```python
from build123d import *

# Parameters (mm, degrees)
SKETCH1_R                = 18.5
BOSS_EXTRUDE1_DEPTH      = 5
SKETCH2_R                = 6.2
CUT_EXTRUDE1_DEPTH       = 10
SKETCH3_R                = 1.6999999999999995
SKETCH3_R_2              = 1.6999999999998752
SKETCH3_R_3              = 1.7000000000002367
SKETCH3_R_4              = 1.700000000000381
SKETCH3_R_5              = 1.7000000000003195
SKETCH3_R_6              = 1.7000000000003193
CUT_EXTRUDE2_DEPTH       = 10
BOSS_EXTRUDE2_DEPTH      = 50
BOSS_EXTRUDE3_DEPTH      = 7
CUT_EXTRUDE3_DEPTH       = 20
BOSS_EXTRUDE4_DEPTH      = 8.5
BOSS_EXTRUDE4_DEPTH_BACK = 15.499999999999996
SKETCH7_R                = 3.799999999999999
SKETCH8_R                = 4.000000000000005
SKETCH8_R_2              = 1.7500000000000004
SKETCH8_R_3              = 4.000000000000007
BOSS_EXTRUDE5_DEPTH      = 4
CUT_EXTRUDE4_START       = -2
SKETCH8_2_R              = 1.7500000000000004
CUT_EXTRUDE4_DEPTH       = 2
FILLET1_R                = 5
SKETCH9_R                = 3.0000000000000036
CUT_EXTRUDE5_DEPTH       = 2.5
CUT_EXTRUDE6_DEPTH       = 182.00138122207798
FILLET2_R                = 10
SKETCH11_W               = 22.00000000000001
SKETCH11_H               = 61.99999999999998
CUT_EXTRUDE7_DEPTH       = 182.00138122207798
FILLET3_R                = 5


with BuildPart() as part:
    # Sketch1 → Boss-Extrude1 (new body)
    with BuildSketch(Plane(origin=(0, 0, 0), x_dir=(0, 0, -1), z_dir=(1, 0, 0))):
        Circle(SKETCH1_R)
    extrude(amount=BOSS_EXTRUDE1_DEPTH)

    # Sketch2 → Cut-Extrude1 (cut)
    with BuildSketch(Plane(origin=(5, 0, 0), x_dir=(0, 0, -1), z_dir=(1, 0, 0))):
        with Locations((0, 7)):
            Circle(SKETCH2_R)
    extrude(amount=-CUT_EXTRUDE1_DEPTH, mode=Mode.SUBTRACT)

    # Sketch3 → Cut-Extrude2 (cut)
    with BuildSketch(Plane(origin=(0, 0, 0), x_dir=(0, 0, -1), z_dir=(1, 0, 0))):
        with Locations((15.5, 0)):
            Circle(SKETCH3_R)
        with Locations((7.750000000000335, -13.423393758658609)):
            Circle(SKETCH3_R_2)
        with Locations((-7.749999999999674, -13.423393758658612)):
            Circle(SKETCH3_R_3)
        with Locations((-15.499999999999568, 0)):
            Circle(SKETCH3_R_4)
        with Locations((-7.749999999999682, 13.42339375865861)):
            Circle(SKETCH3_R_5)
        with Locations((7.749999999999989, 13.42339375865842)):
            Circle(SKETCH3_R_6)
    extrude(amount=CUT_EXTRUDE2_DEPTH, mode=Mode.SUBTRACT)

    # Sketch4 → Boss-Extrude2 (add)
    with BuildSketch(Plane.ZY):
        with BuildLine():
            Line((-18.5, 0), (-21.5, 0))
            ThreePointArc((-21.5, 0), (-3.95e-15, -21.5), (21.5, 0))
            Line((21.5, 0), (18.5, 0))
            ThreePointArc((18.5, 0), (-3.4e-15, -18.5), (-18.5, 0))
        make_face()
    extrude(amount=-BOSS_EXTRUDE2_DEPTH)

    # Sketch5 → Boss-Extrude3 (add)
    with BuildSketch(Plane.ZY):
        with BuildLine():
            Line((-21.5, 0), (-18.5, 0))
            ThreePointArc((-18.5, 0), (-3.4e-15, -18.5), (18.5, 0))
            Line((18.5, 0), (21.5, 0))
            Line((21.5, 0), (21.500000000000018, -174.5))
            Line((21.500000000000018, -174.5), (-21.49999999999998, -174.5))
            Line((-21.49999999999998, -174.5), (-21.5, 0))
        make_face()
    extrude(amount=-BOSS_EXTRUDE3_DEPTH)

    # Sketch6 → Cut-Extrude3 (cut)
    with BuildSketch(Plane(origin=(7, 0, 0), x_dir=(0, 0, -1), z_dir=(1, 0, 0))):
        with BuildLine():
            ThreePointArc((2.57571e-12, -174.5), (-15.202795795509834, -168.2027957955117), (-21.499999999999957, -153.00000000000003))
            Line((-21.500000000000014, -153.00000000000003), (-21.500000000000018, -174.5))
            Line((-21.500000000000018, -174.5), (2.57572e-12, -174.5))
        make_face()
        with BuildLine():
            Line((21.49999999999998, -174.5), (21.499999999999982, -153.00000000000003))
            ThreePointArc((21.5, -153.00000000000003), (15.20279579551168, -168.20279579550987), (2.57571e-12, -174.5))
            Line((2.57572e-12, -174.5), (21.499999999999982, -174.5))
        make_face()
    extrude(amount=-CUT_EXTRUDE3_DEPTH, mode=Mode.SUBTRACT)

    # Sketch7 → Boss-Extrude4 (add, two sides: drawn at the far end of the back side and taken through both)
    with BuildSketch(Plane(origin=(7, 0, 0), x_dir=(0, 0, -1), z_dir=(1, 0, 0)).offset(-BOSS_EXTRUDE4_DEPTH_BACK)):
        with Locations((2.082e-14, -153.00000000000003)):
            Circle(SKETCH7_R)
    extrude(amount=BOSS_EXTRUDE4_DEPTH + BOSS_EXTRUDE4_DEPTH_BACK)

    # Sketch8 → Boss-Extrude5 (add)
    # profile 1 of 4: a face of its own
    with BuildSketch(Plane(origin=(7, 0, 0), x_dir=(0, 0, -1), z_dir=(1, 0, 0))):
        with Locations(Location((10.160000000000018, -121.88999999999999, 0), (0, 0, 180))):
            Circle(SKETCH8_R)
        with Locations((10.160000000000018, -121.88999999999999)):
            Circle(SKETCH8_R_2, mode=Mode.SUBTRACT)
    # profile 2 of 4: a face of its own
    with BuildSketch(Plane(origin=(7, 0, 0), x_dir=(0, 0, -1), z_dir=(1, 0, 0))):
        with Locations(Location((-10.159999999999984, -121.88999999999999, 0), (0, 0, 180))):
            Circle(SKETCH8_R_3)
        with Locations((-10.159999999999984, -121.88999999999999)):
            Circle(SKETCH8_R_2, mode=Mode.SUBTRACT)
    # profile 3 of 4: a face of its own
    with BuildSketch(Plane(origin=(7, 0, 0), x_dir=(0, 0, -1), z_dir=(1, 0, 0))):
        with Locations(Location((-10.159999999999984, -104.10999999999999, 0), (0, 0, 180))):
            Circle(SKETCH8_R_3)
        with Locations((-10.159999999999984, -104.10999999999999)):
            Circle(SKETCH8_R_2, mode=Mode.SUBTRACT)
    # profile 4 of 4: a face of its own
    with BuildSketch(Plane(origin=(7, 0, 0), x_dir=(0, 0, -1), z_dir=(1, 0, 0))):
        with Locations(Location((10.160000000000018, -104.10999999999999, 0), (0, 0, 180))):
            Circle(SKETCH8_R)
        with Locations((10.160000000000018, -104.10999999999999)):
            Circle(SKETCH8_R_2, mode=Mode.SUBTRACT)
    extrude(amount=BOSS_EXTRUDE5_DEPTH)

    # Sketch8_2 → Cut-Extrude4 (cut)
    with BuildSketch(Plane(origin=(7, 0, 0), x_dir=(0, 0, -1), z_dir=(1, 0, 0)).offset(CUT_EXTRUDE4_START)):
        with Locations((-10.159999999999984, -121.88999999999999)):
            Circle(SKETCH8_2_R)
        with Locations((-10.159999999999984, -104.10999999999999)):
            Circle(SKETCH8_2_R)
        with Locations((10.160000000000018, -104.10999999999999)):
            Circle(SKETCH8_2_R)
        with Locations((10.160000000000018, -121.88999999999999)):
            Circle(SKETCH8_2_R)
    extrude(amount=CUT_EXTRUDE4_DEPTH, mode=Mode.SUBTRACT)

    # Fillet1
    fillet1_edges = [part.edges().sort_by_distance(p)[0] for p in [
        (7, -21.5, -2.2e-15),
    ]]
    fillet(fillet1_edges, radius=FILLET1_R)

    # Sketch9 → Cut-Extrude5 (cut)
    with BuildSketch(Plane(origin=(15.5, 0, 0), x_dir=(0, 0, -1), z_dir=(1, 0, 0))):
        with Locations((2.082e-14, -153.00000000000003)):
            Circle(SKETCH9_R)
    extrude(amount=-CUT_EXTRUDE5_DEPTH, mode=Mode.SUBTRACT)

    # Sketch10 → Cut-Extrude6 (cut, through all)
    with BuildSketch(Plane(origin=(7, 0, 0), x_dir=(0, 0, -1), z_dir=(1, 0, 0))):
        with BuildLine():
            Line((-15.000000000000016, -137.57296518391348), (-15.000000000000014, -21.84605227495347))
            ThreePointArc((-15.000000000000018, -21.84605227495347), (-18.524475882395627, -18.94977026991469), (-21.5, -15.491933384829668))
            Line((-21.5, -15.491933384829668), (-21.5, -152.13779166279446))
            ThreePointArc((-21.500000000000007, -152.13779166279446), (-19.64932677192729, -144.23088598393383), (-15.000000000000014, -137.57296518391348))
        make_face()
        with BuildLine():
            ThreePointArc((21.499999999999996, -15.491933384829675), (18.52447588239562, -18.949770269914705), (14.999999999999996, -21.846052274953482))
            Line((14.999999999999996, -21.846052274953482), (14.999999999999995, -137.57296518391342))
            ThreePointArc((14.999999999999995, -137.57296518391342), (19.649326771927107, -144.23088598393335), (21.499999999999993, -152.1377916627935))
            Line((21.499999999999996, -152.1377916627935), (21.499999999999996, -15.491933384829672))
        make_face()
    extrude(amount=-CUT_EXTRUDE6_DEPTH, mode=Mode.SUBTRACT)

    # Fillet2
    fillet2_edges = [part.edges().sort_by_distance(p)[0] for p in [
        (3.5, -137.57296518391348, 15.000000000000014),
        (3.5, -137.57296518391342, -14.999999999999991),
        (3.5, -21.846052274953486, -14.999999999999998),
        (3.5, -15.491933384829675, -21.5),
        (3.5, -21.846052274953465, 15.000000000000014),
        (3.5, -15.491933384829668, 21.5),
    ]]
    fillet(fillet2_edges, radius=FILLET2_R)

    # Sketch11 → Cut-Extrude7 (cut, through all)
    with BuildSketch(Plane(origin=(7, 0, 0), x_dir=(0, 0, -1), z_dir=(1, 0, 0))):
        with Locations((-8.88e-15, -61.47322598734716)):
            Rectangle(SKETCH11_W, SKETCH11_H)
    extrude(amount=-CUT_EXTRUDE7_DEPTH, mode=Mode.SUBTRACT)

    # Fillet3
    fillet3_edges = [part.edges().sort_by_distance(p)[0] for p in [
        (3.5, -30.47322598734717, -10.999999999999996),
        (3.5, -92.47322598734716, -10.999999999999996),
        (3.5, -92.47322598734716, 11.000000000000014),
        (3.5, -30.47322598734717, 11.000000000000014),
    ]]
    fillet(fillet3_edges, radius=FILLET3_R)


solid = part.part
```
The model under review builds one solid part; all positions refer to its coordinate system, in mm. A direction names the side the tool comes from. Round coordinates to 2 decimals unless told otherwise and drop trailing zeros. Order: outer loops, then holes, each group sorted by start corner. A loop starts at its lowest first (then second) coordinate and runs counter-clockwise, first axis right, second up.
Item 1: Machinability: for faces 4 (the cylindrical face through (3.451, -136.98, 15.516)), 5 (the flat face through (4, -92.473, 0)), 6 (the flat face through (11, -102, 11)), 7 (the flat face through (50, -19, 0)), 8 (the flat face through (5, -122, 10)), which of the approach directions +Z, -Z, +X, -X, +Y, -Y give a long, thin tool a straight path to every point of the face, cutting with its end or side? Answer none if there is none.
Working result:
face 4: +Z, +X, -X
face 5: +X, -X
face 6: +Z, -Z, +X, -Y
face 7: +Z, -Z, +X, +Y, -Y
face 8: +X
Item 2: Add section C-C, the plane y = 5. State the section outline as (x, z) points, and give its area (3 significant figures).
Working result:
outline: (0, -17.81) - (5, -17.81) - (5, -5.87) - (0, -5.87) - close; (0, 5.87) - (5, 5.87) - (5, 17.81) - (0, 17.81) - close
area: 119 mm2
Item 3: Draft analysis for pull direction Y (two halves, no side actions). For faces 1 (the cylindrical face through (-4.31, -156.71, 0.82)), 2 (the flat face through (11, -102, -9)), 3 (the cylindrical face through (2.465, -14.075, 6.18)), state which applies: released by +Y, released by -Y, zero draft, split by the parting line, or undercut.
Working result:
face 1: split by the parting line
face 2: zero draft
face 3: undercut
Item 4: For pin 1 (6.5 mm diameter, centred on y = -153, z = -0.5, fed in from +X); pin 2 (6 mm diameter, centred on x = 10.5, z = 10.5, fed in from -Y); pin 3 (1.5 mm diameter, centred on y = -110.5, z = 3.5, fed in from +X), all flat-tipped, find the tip position at first contact; note any pin that passes through.
Working result:
pin 1: stops at x = 15.5
pin 2: stops at y = -125.89
pin 3: stops at x = 7
Item 5: Add section B-B, the plane z = 0. Count the separate pieces of the cut face and the enclosed holes in it, and give its area (3 significant figures).
Working result:
separate pieces: 3
enclosed holes: 0
area: 1,030 mm2
Item 6: To check wall thickness, follow probe 1 along Y at (x, z) = (14.75, 0); probe 2 along Y at (x, z) = (3.05, 7.75); probe 3 along Y at (x, z) = (3, 7). State the ranges of each line that lie inside material, in increasing order.
Working result:
probe 1: y = -156.8 to -156, -150 to -149.2, -21.5 to -18.5
probe 2: y = -173.05 to -92.16, -30.79 to -15.12, -11.72 to 11.72, 15.12 to 16.8
probe 3: y = -173.33 to -92.37, -30.57 to -14.95, -11.9 to 11.9, 14.95 to 17.12
Item 7: Add section A-A, the plane y = -43. State the section outline as (x, z) points.
Working result:
outline: (0, -15) - (7, -15) - (7, -11) - (0, -11) - close; (0, 11) - (7, 11) - (7, 15) - (0, 15) - close
Item 8: Add section D-D, the plane y = -121.89. State the section outline as (x, z) points.
Working result:
outline: (0, -15) - (7, -15) - (7, -14.16) - (11, -14.16) - (11, -11.91) - (5, -11.91) - (5, -8.41) - (11, -8.41) - (11, -6.16) - (7, -6.16) - (7, 6.16) - (11, 6.16) - (11, 8.41) - (5, 8.41) - (5, 11.91) - (11, 11.91) - (11, 14.16) - (7, 14.16) - (7, 15) - (0, 15) - close
